Verification items for this drawing (mm, ordinates from the low corner). Give positions to 0.01 mm unless a question says otherwise; leave off trailing zeros. Loops run counter-clockwise (first coordinate to the right, second up) from the corner with the lowest first, then second, coordinate; pieces in that order, holes last. Notation, with made-up numbers: M 43,-21.5 L 60,-21.5 A18 ccw 60,2.5 Z; hole C 28,86 d3. An arc over 180 degrees is marked long. Answer in a Markdown table with one row per item.
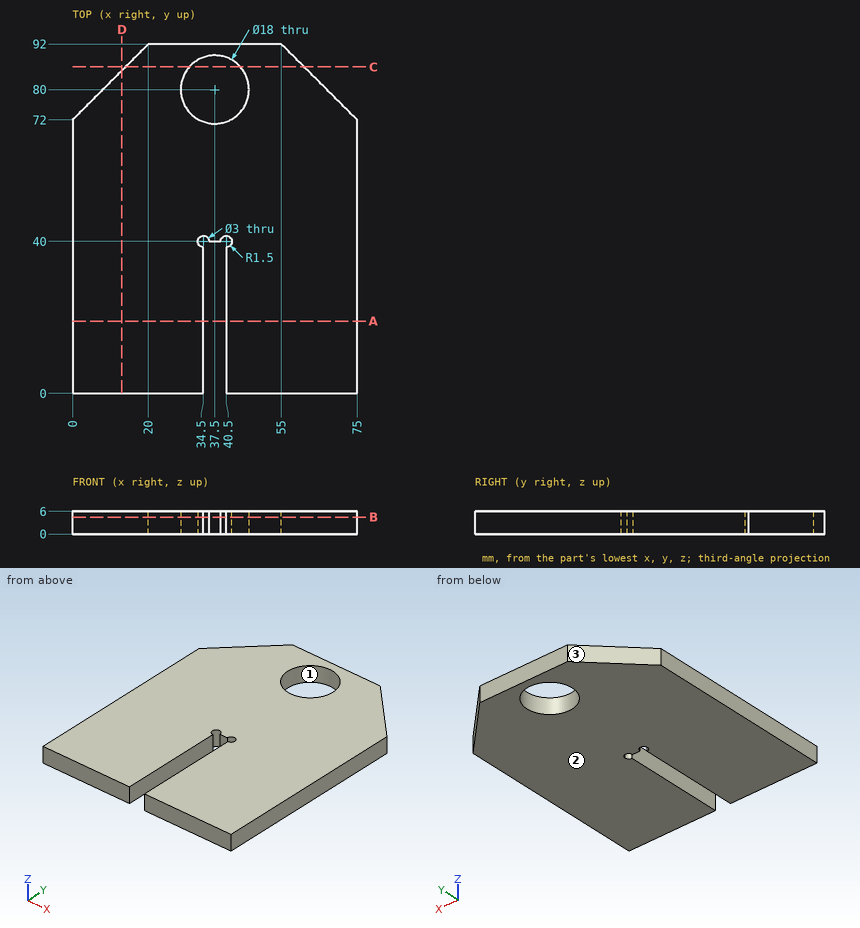
Item 1: Go/stop test with flat-tipped pins: pin 1 (23.5 mm diameter, centred on x = 37.5, y = 80, fed in from +Z); pin 2 (0.9 mm diameter, centred on x = 37, z = 2, fed in from -Y). Record where each tip stops, or that it passes through.
Reported:
| item | result |
|---|---|
| pin 1 | stops at z = 6 |
| pin 2 | stops at y = 40 |
Item 2: Sectioned sample at D-D (x = 13). Record the cut outline in (y, z), and give its area (3 significant figures).
Reported:
| item | result |
|---|---|
| outline | M 0,0 L 85,0 L 85,6 L 0,6 Z |
| area | 510 mm^2 |
Item 3: Sectioned sample at A-A (y = 19). Record the cut outline in (x, z).
Reported:
| item | result |
|---|---|
| outline | M 0,0 L 34.5,0 L 34.5,6 L 0,6 Z; M 40.5,0 L 75,0 L 75,6 L 40.5,6 Z |
Item 4: Sectioned sample at C-C (y = 86). Record the cut outline in (x, z).
Reported:
| item | result |
|---|---|
| outline | M 14,0 L 30.79,0 L 30.79,6 L 14,6 Z; M 44.21,0 L 61,0 L 61,6 L 44.21,6 Z |
Item 5: Sectioned sample at B-B (z = 4.45). Record the cut outline in (x, y), and give its area (4 significant figures).
Reported:
| item | result |
|---|---|
| outline | M 0,0 L 34.5,0 L 34.5,38.5 A1.5 cw long 36,40 L 39,40 A1.5 cw long 40.5,38.5 L 40.5,0 L 75,0 L 75,72 L 55,92 L 20,92 L 0,72 Z; hole C 37.5,80 d18 |
| area | 5,995 mm^2 |
Item 6: Release check for a two-part mould opening along Y. For the marked faces 1, 2 and 3 record: released by +Y, released by -Y, zero draft, split by the parting line, or undercut.
Reported:
| item | result |
|---|---|
| face 1 | undercut |
| face 2 | zero draft |
| face 3 | released by +Y |
Item 7: Scan lines: L1, parallel to X at y = 10.5, z = 1.25; L2, parallel to X at y = 84, z = 1.9; L3, parallel to Y at x = 30, z = 1.4 (1 decimal). Record each from-to range of solid material in increasing order. Write a range as [from, to].
Reported:
| item | result |
|---|---|
| L1 | x = [0, 34.5], [40.5, 75] |
| L2 | x = [12, 29.44], [45.56, 63] |
| L3 | y = [0, 75], [85, 92] |
